Part model, mm, in its own coordinate system. Round coordinates to 2 decimals unless told otherwise and drop trailing zeros. Write each loop counter-clockwise with the first axis right and the second up, starting at its lowest first coordinate (ties: lowest second). Pieces come first, ordered by that corner, then holes. Notation, with made-up numbers: M 37.25,29 L 44.25,29 A11 ccw 44.25,47 Z; hole C -25.75,10 d7. An arc over 180 degrees is marked long. Answer as a JSON object with one key per item and string values. Group by question number.
1. Band-saw the part on A-A, the plane x = 0. Write the cut outline in (y, z).
2. Drop a flat-ended pin along its axis: pin 1 (1.8 mm diameter, centred on x = -30.5, y = 44, fed in from -Z) (3 decimals). Give the stop position or say it passes through.
3. Band-saw the part on B-B, the plane z = 0.15. Write the cut outline in (x, y), plus the area to 4 significant figures.
4. Drill centre lines: line 1 (Y direction, x = -30.5, z = 0.6); line 2 (Y direction, x = 3.5, z = 0.75); line 3 (X direction, y = 4, z = 0.95). Where is each one in solid material? Low to high. Write a range as from..to.
5. Band-saw the part on C-C, the plane y = 44. Write the cut outline in (x, z), plus the area to 3 significant figures.
6. Band-saw the part on D-D, the plane x = -30.5. Write the cut outline in (y, z), plus the area to 3 significant figures.
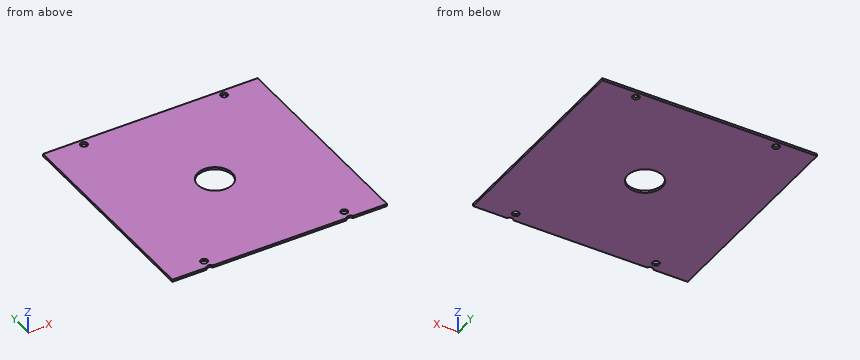
from build123d import *

# Parameters (mm, degrees)
SKETCH1_W                    = 93.4
SKETCH1_H                    = 93.4
BOSS_EXTRUDE1_DEPTH          = 1
F_3_0_3_DIAMETER_HOLE1_D     = 3
F_3_0_3_DIAMETER_HOLE1_DEPTH = 1
SKETCH_1_R                   = 7.5
CUT_EXTRUDE_1_DEPTH          = 67.051343665


with BuildPart() as part:
    # Sketch1 → Boss-Extrude1 (new body)
    with BuildSketch(Plane.XY):
        Rectangle(SKETCH1_W, SKETCH1_H)
    extrude(amount=BOSS_EXTRUDE1_DEPTH)

    # Ø3.0 (3) Diameter Hole1
    with Locations(Plane.XY.offset(1)):
        with Locations((-30.5, -47.3), (30.5, -47.3), (30.5, -42.7), (-30.5, -42.7), (-30.5, 44), (30.5, 44), (-30.5, -66), (30.5, -66)):
            Hole(F_3_0_3_DIAMETER_HOLE1_D / 2, depth=F_3_0_3_DIAMETER_HOLE1_DEPTH)

    # Эскиз1 → Вырез-Вытянуть1 (cut, through all)
    with BuildSketch(Plane.XY.offset(1)):
        Circle(SKETCH_1_R)
    extrude(amount=-CUT_EXTRUDE_1_DEPTH, mode=Mode.SUBTRACT)


solid = part.part
Worked answers:
{
 "1": {"outline": "M -46.7,0 L -7.5,0 L -7.5,1 L -46.7,1 Z; M 7.5,0 L 46.7,0 L 46.7,1 L 7.5,1 Z"},
 "2": {"pin 1": "passes through"},
 "3": {"outline": "M -46.7,-46.7 L -31.87,-46.7 A1.5 cw -29.13,-46.7 L 29.13,-46.7 A1.5 cw 31.87,-46.7 L 46.7,-46.7 L 46.7,46.7 L -46.7,46.7 Z; hole C -30.5,-42.7 d3; hole C -30.5,44 d3; hole C 0,0 d15; hole C 30.5,-42.7 d3; hole C 30.5,44 d3", "area": "8,515 mm^2"},
 "4": {"line 1": "y = -45.8..-44.2, -41.2..42.5, 45.5..46.7", "line 2": "y = -46.7..-6.63, 6.63..46.7", "line 3": "x = -46.7..-6.34, 6.34..46.7"},
 "5": {"outline": "M -46.7,0 L -32,0 L -32,1 L -46.7,1 Z; M -29,0 L 29,0 L 29,1 L -29,1 Z; M 32,0 L 46.7,0 L 46.7,1 L 32,1 Z", "area": "87.4 mm^2"},
 "6": {"outline": "M -45.8,0 L -44.2,0 L -44.2,1 L -45.8,1 Z; M -41.2,0 L 42.5,0 L 42.5,1 L -41.2,1 Z; M 45.5,0 L 46.7,0 L 46.7,1 L 45.5,1 Z", "area": "86.5 mm^2"}
}
